Source: CAD feature listing. Evaluate the final solid. Frame: model axes, mm. Coordinates: 2 decimals unless noted, no trailing zeros. Order: outer loops, then holes, each group sorted by start corner. A loop starts at its lowest first (then second) coordinate and runs counter-clockwise, first axis right, second up.
Item 1: Section B-B on z = 63.5. Return the cut outline in (x, y), then the cut area to 3 significant figures.
Item 2: Section C-C on y = 1.85. State how many separate pieces and enclosed holes the cut face has, then the cut area to 3 significant figures.
Item 3: Contact query for flat-ended pins moving along their axis: P1, Ø6, axis at x = 63.5, z = 63.5, coming from the -Y side; P2, Ø10, axis at x = -36.5, z = -38.5, coming from the -Y side. Output: stop coordinate, or through.
Item 4: Ray query, line 1 (X direction, y = 1.6, z = -63.5); line 2 (Z direction, x = 2, y = 4.55); line 3 (Z direction, x = 60.5, y = 2.4). Return the intervals inside material, ascending.
Item 5: Mould query, pull axis X, two halves, no side actions, for faces 1 (the flat face through (-76.2, 2, 1)), 2 (the flat face through (1, 2, 76.2)), 3 (the cylindrical face through (74.39, 2.46, 74.29)), 4 (the cylindrical face through (-0.07, 2.46, 60.35)). Classes: released by +X, released by -X, zero draft, split by the parting line, or undercut.
Item 6: Section A-A on x = 63.5. Return the cut outline in (y, z).
from build123d import *

# Parameters (mm, degrees)
SKETCH1_R           = 3.302
BOSS_EXTRUDE1_DEPTH = 5
SKETCH2_R           = 1.05
CUT_EXTRUDE2_DEPTH  = 108.879006299


with BuildPart() as part:
    # Sketch1 → Boss-Extrude1 (new body)
    with BuildSketch(Plane(origin=(0, 0, 0), x_dir=(1, 0, 0), z_dir=(0, 1, 0))):
        with BuildLine():
            Line((-69.85, 76.2), (69.85, 76.2))
            ThreePointArc((69.85, 76.2), (74.340128061, 74.340128061), (76.2, 69.85))
            Line((76.2, 69.85), (76.2, -69.85))
            ThreePointArc((76.2, -69.85), (74.340128061, -74.340128061), (69.85, -76.2))
            Line((69.85, -76.2), (-69.85, -76.2))
            ThreePointArc((-69.85, -76.2), (-74.340128061, -74.340128061), (-76.2, -69.85))
            Line((-76.2, -69.85), (-76.2, 69.85))
            ThreePointArc((-76.2, 69.85), (-74.340128061, 74.340128061), (-69.85, 76.2))
        make_face()
        with Locations(Location((63.5, 63.5, 0), (0, 0, 270))):
            Circle(SKETCH1_R, mode=Mode.SUBTRACT)
        with Locations(Location((63.5, -63.5, 0), (0, 0, 90))):
            Circle(SKETCH1_R, mode=Mode.SUBTRACT)
        with Locations(Location((-63.5, -63.5, 0), (0, 0, 270))):
            Circle(SKETCH1_R, mode=Mode.SUBTRACT)
        with Locations(Location((-63.5, 63.5, 0), (0, 0, 90))):
            Circle(SKETCH1_R, mode=Mode.SUBTRACT)
        with Locations(Location((0, 0, 0), (0, 0, 270))):
            Circle(SKETCH1_R, mode=Mode.SUBTRACT)
    extrude(amount=BOSS_EXTRUDE1_DEPTH)

    # Sketch2 → Cut-Extrude2 (cut, through all)
    with BuildSketch(Plane(origin=(0, 0, 0), x_dir=(1, 0, 0), z_dir=(0, 1, 0))):
        with Locations(Location((0, -42.125, 0), (0, 0, 270))):
            Circle(SKETCH2_R)
        with Locations(Location((0, -70.375, 0), (0, 0, 270))):
            Circle(SKETCH2_R)
        with BuildLine():
            Line((-3.2, -56.110367219), (-3.2, -57.15))
            ThreePointArc((-3.2, -57.15), (0, -60.35), (3.2, -57.15))
            Line((3.2, -57.15), (3.2, -56.110367219))
            ThreePointArc((3.2, -56.110367219), (0, -44.6), (-3.2, -56.110367219))
        make_face()
    extrude(amount=CUT_EXTRUDE2_DEPTH, mode=Mode.SUBTRACT)


solid = part.part
Answer list:
1. outline: (-76.2, 0) - (-66.8, 0) - (-66.8, 5) - (-76.2, 5) - close; (-60.2, 0) - (60.2, 0) - (60.2, 5) - (-60.2, 5) - close; (66.8, 0) - (76.2, 0) - (76.2, 5) - (66.8, 5) - close
1. area: 696 mm2
2. separate pieces: 1
2. enclosed holes: 8
2. area: 22,900 mm2
3. P1: passes through
3. P2: stops at y = 0
4. line 1: x = -76.2 to -66.8, -60.2 to 60.2, 66.8 to 76.2
4. line 2: z = -76.2 to -2.63, 2.63 to 44.93, 59.65 to 76.2
4. line 3: z = -76.2 to -64.88, -62.12 to 62.12, 64.88 to 76.2
5. face 1: released by -X
5. face 2: zero draft
5. face 3: released by +X
5. face 4: undercut
6. outline: (0, -76.2) - (5, -76.2) - (5, -66.8) - (0, -66.8) - close; (0, -60.2) - (5, -60.2) - (5, 60.2) - (0, 60.2) - close; (0, 66.8) - (5, 66.8) - (5, 76.2) - (0, 76.2) - close
